For this review, take the finished solid that the model builds, in its own axes (mm). A direction names the side the tool comes from. Round coordinates to 2 decimals unless told otherwise and drop trailing zeros. Write each loop counter-clockwise with the first axis right and the second up, starting at its lowest first coordinate (ties: lowest second). Pieces come first, ordered by that corner, then holes. Notation, with made-up numbers: (-29.5, -27.5) - (0.5, -27.5) arc R27 cw to (0.5, 8.5) - close; hole circle Ø10 at (-26.5, 46.5). An arc over 180 degrees is marked (long way). One line per item, written item: value. Start each with the question number.
Q1. For probe 1 along Y at (x, z) = (11.43, 12.25); probe 2 along Y at (x, z) = (4.75, 4), list the stretches that pass through material, from the lowest coordinate up.
Q2. Clearance check with flat-ended pins moving along their axes: pin 1 Ø1.3 at (x, y) = (11.5, -11.5) entering from +Z; pin 2 Ø6 at (x, y) = (-3, -4.5) entering from +Z. State where each tip first meets the part, or that it passes through.
Q3. Add section B-B on x = -3.25. Write out the cut boundary in (y, z), and give its area (3 significant figures).
Q4. Mouldability with a two-part tool opening along X and no side actions: class faces 1 (the face through (-10.16, 0, 1)), 2 (the face through (12.7, 0, 0)), 3 (the face through (0, 12.7, 0)) as +X half, -X half, draft (parallel to the pull), parting line (faces both ways), or undercut.
Q5. Tool access review of faces 4 (the face through (0, 0, -12.7)), 5 (the face through (0, -10.16, 1)): name each direction out of +Z, -Z, +X, -X, +Y, -Y from which nothing blocks a thin tool from reaching the whole face with its end or side.
Q6. Add section A-A on z = -6. Write out the cut boundary in (x, y).
```python
from build123d import *

# Parameters (mm, degrees)
F1_DEPTH = 12.7
F2_T     = -2.54
F3_R     = 0.8255
F4_DEPTH = 1.27


with BuildPart() as f1:
    # F0 (on Front) → F1 (new body, symmetric)
    with BuildSketch(Plane.XZ):
        Polygon((-12.7, -12.7), (0, -12.7), (12.7, -12.7), (12.7, 0), (12.7, 12.7), (0, 12.7), (-12.7, 12.7), (-12.7, 0), align=None)
    extrude(amount=F1_DEPTH, both=True)

    # F2
    f2_openings = [f1.faces().sort_by_distance(p)[0] for p in [
        (0, 0, 12.7),
    ]]
    offset(amount=F2_T, openings=f2_openings)

    # F3 (on face) → F4 (cut)
    with BuildSketch(Plane.XY.offset(12.7)):
        with Locations((-11.43, 11.43)):
            Circle(F3_R)
        with Locations((11.43, 11.43)):
            Circle(F3_R)
        with Locations((11.43, -11.43)):
            Circle(F3_R)
        with Locations((-11.43, -11.43)):
            Circle(F3_R)
    extrude(amount=-F4_DEPTH, mode=Mode.SUBTRACT)


solid = f1.part
```
Result set:
1. probe 1: y = -12.7 to -12.26, -10.6 to 10.6, 12.26 to 12.7
1. probe 2: y = -12.7 to -10.16, 10.16 to 12.7
2. pin 1: stops at z = 11.43
2. pin 2: stops at z = -10.16
3. outline: (-12.7, -12.7) - (12.7, -12.7) - (12.7, 12.7) - (10.16, 12.7) - (10.16, -10.16) - (-10.16, -10.16) - (-10.16, 12.7) - (-12.7, 12.7) - close
3. area: 181 mm^2
4. face 1: undercut
4. face 2: +X half
4. face 3: draft
5. face 4: -Z, +X, -X, +Y, -Y
5. face 5: +Z
6. outline: (-12.7, -12.7) - (12.7, -12.7) - (12.7, 12.7) - (-12.7, 12.7) - close; hole (-10.16, -10.16) - (10.16, -10.16) - (10.16, 10.16) - (-10.16, 10.16) - close
